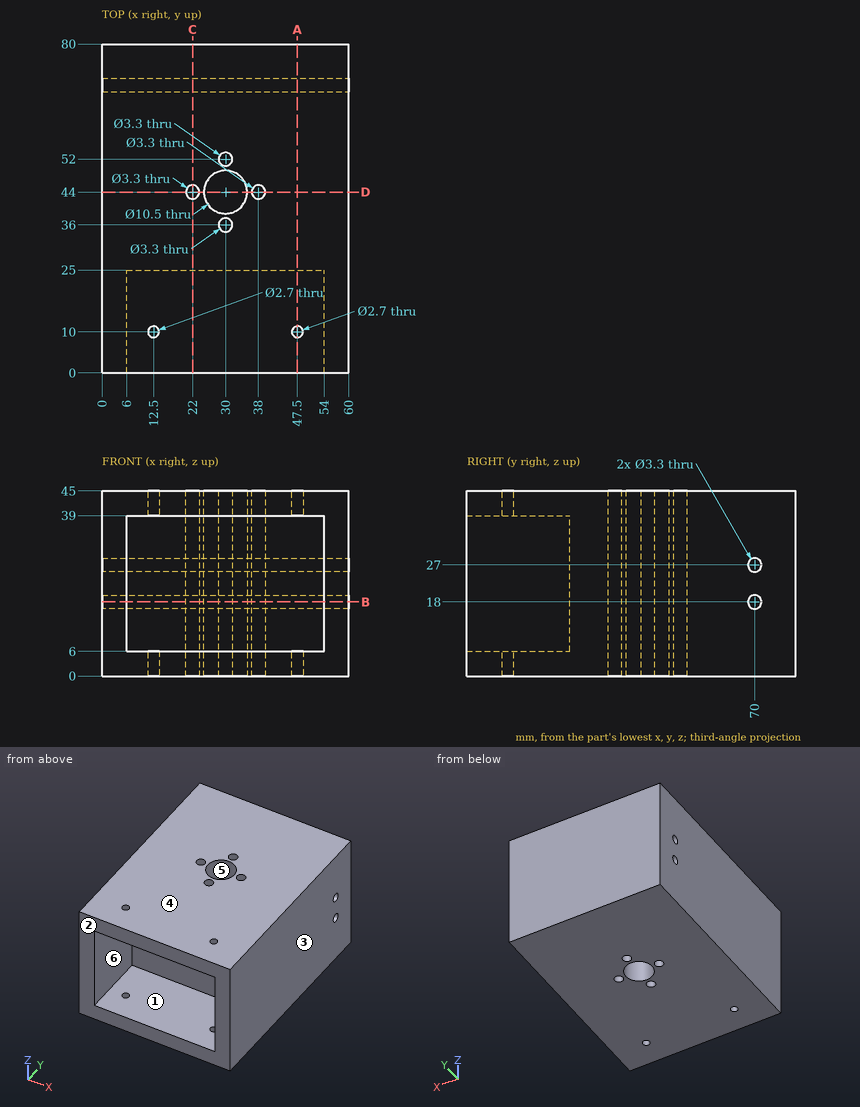
Could you check a few things on this drawing? It's one solid part, dimensions in mm from its lowest x, y, z. A direction names the side the tool comes from. Give positions to 0.01 mm unless a question says otherwise; leave off trailing zeros. Loops run counter-clockwise (first coordinate to the right, second up) from the corner with the lowest first, then second, coordinate; pieces in that order, holes last. Notation, with made-up numbers: (-10.75, -15.75) -> (42.25, -15.75) arc R13 ccw to (42.25, -7.75) -> close; hole circle Ø8 at (6.25, -38). An arc over 180 degrees is marked (long way). Use one line per item in the form item = value. Start each with the question number.
1) Thinking about a two-plate mould opening in X: for the marked faces 3, 4, 5 and 6, which applies, +X half, -X half, draft (parallel to the pull), parting line (faces both ways), or undercut?
2) Which directions (+Z, -Z, +X, -X, +Y, -Y) give clear straight access to the entire face, cutting with the end or side of a thin tool? Please do the marked faces 1 and 2.
3) Imagine slicing it at D-D (y = 44). Please give me the cut outline in (x, z).
4) Imagine slicing it at B-B (z = 18). Please give me the cut outline in (x, y).
5) Imagine slicing it at A-A (x = 47.5). Please give me the cut outline in (y, z).
6) Imagine slicing it at C-C (x = 22). Please give me the cut outline in (y, z).
7) Please list where these lines run through material, in increasing order: line 1 along Y through (x, z) = (30, 21.5); line 2 along Y through (x, z) = (14, 18); line 3 along Y through (x, z) = (38, 13).
Check values:
q1.face_3 = +X half
q1.face_4 = draft
q1.face_5 = undercut
q1.face_6 = undercut
q2.face_1 = -Y
q2.face_2 = +Z, -Z, +X, -X, -Y
q3.outline = (0, 0) -> (20.35, 0) -> (20.35, 45) -> (0, 45) -> close; (23.65, 0) -> (24.75, 0) -> (24.75, 45) -> (23.65, 45) -> close; (35.25, 0) -> (36.35, 0) -> (36.35, 45) -> (35.25, 45) -> close; (39.65, 0) -> (60, 0) -> (60, 45) -> (39.65, 45) -> close
q4.outline = (0, 0) -> (6, 0) -> (6, 25) -> (54, 25) -> (54, 0) -> (60, 0) -> (60, 68.35) -> (0, 68.35) -> close; (0, 71.65) -> (60, 71.65) -> (60, 80) -> (0, 80) -> close; hole circle Ø3.3 at (22, 44); hole circle Ø10.5 at (30, 44); hole circle Ø3.3 at (30, 36); hole circle Ø3.3 at (30, 52); hole circle Ø3.3 at (38, 44)
q5.outline = (0, 0) -> (8.65, 0) -> (8.65, 6) -> (0, 6) -> close; (0, 39) -> (8.65, 39) -> (8.65, 45) -> (0, 45) -> close; (11.35, 0) -> (80, 0) -> (80, 45) -> (11.35, 45) -> (11.35, 39) -> (25, 39) -> (25, 6) -> (11.35, 6) -> close; hole circle Ø3.3 at (70, 18); hole circle Ø3.3 at (70, 27)
q6.outline = (0, 0) -> (42.35, 0) -> (42.35, 45) -> (0, 45) -> (0, 39) -> (25, 39) -> (25, 6) -> (0, 6) -> close; (45.65, 0) -> (80, 0) -> (80, 45) -> (45.65, 45) -> close; hole circle Ø3.3 at (70, 18); hole circle Ø3.3 at (70, 27)
q7.line_1 = 25 to 34.35, 37.65 to 38.75, 49.25 to 50.35, 53.65 to 80
q7.line_2 = 25 to 68.35, 71.65 to 80
q7.line_3 = 25 to 42.35, 45.65 to 80
